Source: CAD feature listing. Evaluate the final solid. Frame: model axes, mm. A direction names the side the tool comes from. Give positions to 0.01 mm unless a question says otherwise; leave off trailing zeros. Order: outer loops, then holes, each group sorted by start corner. A loop starts at its lowest first (then second) coordinate and runs counter-clockwise, first axis right, second up. Notation, with made-up numbers: (36, 33.25) - (57, 33.25) arc R27 ccw to (57, 68.25) - close; hole circle Ø11 at (35.25, -8). An arc over 180 degrees is marked (long way). Answer as CSV lines item,"result".
```python
from build123d import *

# Parameters (mm, degrees)
SKETCH1_R           = 19
SKETCH1_R_2         = 10
BOSS_EXTRUDE1_DEPTH = 20
BOSS_EXTRUDE2_DEPTH = 30
BOSS_EXTRUDE3_DEPTH = 40
SKETCH2_R           = 5
BOSS_EXTRUDE4_DEPTH = 10


with BuildPart() as part:
    # Sketch1 → Boss-Extrude1 (new body)
    with BuildSketch(Plane(origin=(0, 0, 0), x_dir=(0, 0, -1), z_dir=(1, 0, 0))):
        Circle(SKETCH1_R)
        Circle(SKETCH1_R_2, mode=Mode.SUBTRACT)
    extrude(amount=BOSS_EXTRUDE1_DEPTH)

    # Sketch1_3 → Boss-Extrude2 (add)
    with BuildSketch(Plane(origin=(0, 0, 0), x_dir=(0, 0, -1), z_dir=(1, 0, 0))):
        with BuildLine():
            ThreePointArc((-27, 0), (0, -27), (27, 0))
            Line((27, 0), (19, 0))
            ThreePointArc((19, 0), (0, -19), (-19, 0))
            Line((-19, 0), (-27, 0))
        make_face()
    extrude(amount=BOSS_EXTRUDE2_DEPTH)

    # Sketch1_4 → Boss-Extrude3 (add)
    with BuildSketch(Plane(origin=(0, 0, 0), x_dir=(0, 0, -1), z_dir=(1, 0, 0))):
        with BuildLine():
            ThreePointArc((-27, 0), (0, -27), (27, 0))
            Line((27, 0), (36, 0))
            Line((36, 0), (44, -31))
            Line((44, -31), (44, -36))
            Line((44, -36), (38, -36))
            Line((38, -36), (38, -96))
            Line((38, -96), (18, -96))
            Line((18, -96), (18, -76))
            Line((18, -76), (-18, -76))
            Line((-18, -76), (-18, -96))
            Line((-18, -96), (-38, -96))
            Line((-38, -96), (-38, -36))
            Line((-38, -36), (-44, -36))
            Line((-44, -36), (-44, -31))
            Line((-44, -31), (-36, 0))
            Line((-36, 0), (-27, 0))
        make_face()
    extrude(amount=BOSS_EXTRUDE3_DEPTH)

    # Sketch2 → Boss-Extrude4 (add)
    # profile 1 of 2: a face of its own
    with BuildSketch(Plane.XZ.offset(36)):
        with BuildLine():
            Line((10, -63), (10, -42))
            Line((10, -42), (30, -42))
            Line((30, -42), (30, -63))
            ThreePointArc((30, -63), (20, -73), (10, -63))
        make_face()
        with Locations(Location((20, -63, 0), (0, 0, 270))):
            Circle(SKETCH2_R, mode=Mode.SUBTRACT)
    # profile 2 of 2: a face of its own
    with BuildSketch(Plane.XZ.offset(36)):
        with BuildLine():
            Line((30, 42), (30, 63))
            ThreePointArc((30, 63), (20, 73), (10, 63))
            Line((10, 63), (10, 42))
            Line((10, 42), (30, 42))
        make_face()
        with Locations(Location((20, 63, 0), (0, 0, 90))):
            Circle(SKETCH2_R, mode=Mode.SUBTRACT)
    extrude(amount=-BOSS_EXTRUDE4_DEPTH)


solid = part.part
```
(1) Access query for faces 1 (the flat face through (20, 0, 28)), 2 (the flat face through (20, -8, -8)), 3 (the flat face through (20, -76, 0)), 4 (the flat face through (5, -33, -44)), 5 (the flat face through (20, -66, 38)). Directions: +Z, -Z, +X, -X, +Y, -Y. A direction counts if a zero-diameter tool reaches every point of the face in a straight line with its end or side. Return the directions, or none.
Completed:
face 1,"+Z, +X, -X, +Y"
face 2,"+X, +Y"
face 3,"+X, -X, -Y"
face 4,"-Z, -X, +Y, -Y"
face 5,"+Z, +X, -X, -Y"
(2) Cut plane A-A (z = 0). Return loops of the section in (x, y), then the cut area to 3 significant figures.
Completed:
outline,"(0, -76) - (40, -76) - (40, -27) - (30, -27) - (30, -19) - (20, -19) - (20, -10) - (0, -10) - close; (0, 10) - (20, 10) - (20, 19) - (0, 19) - close"
area,"2,560 mm²"
(3) Contact query for flat-ended pins moving along their axis: pin 1 (10 mm diameter, centred on y = -9.5, z = 18.5, fed in from +X); pin 2 (2 mm diameter, centred on x = 10, z = 58, fed in from +Y); pin 3 (18.5 mm diameter, centred on x = 13, z = 26, fed in from +Y). Output: stop coordinate, or through.
Completed:
pin 1,"x = 30"
pin 2,"y = -26"
pin 3,"y = 8.97"
(4) Ray query, line 1 (X direction, y = -31.75, z = 63); line 2 (Y direction, x = 19, z = 0); line 3 (Z direction, x = 34, y = -86). Return the intervals inside material, ascending. Write a range as from..to.
Completed:
line 1,"10..15, 25..30"
line 2,"-76..-10, 10..19"
line 3,"-38..-18, 18..38"
(5) Mould query, pull axis Z, two halves, no side actions, for faces 6 (the cylindrical face through (20, -31, -73)), 7 (the flat face through (20, 0, -27)), 8 (the cylindrical face through (15.12, -31.07, -61.92)). Classes: released by +Z, released by -Z, zero draft, split by the parting line, or undercut.
Completed:
face 6,"released by -Z"
face 7,"zero draft"
face 8,"undercut"
(6) Cut plane C-C (x = 8). Return loops of the section in (y, z).
Completed:
outline,"(-96, -38) - (-36, -38) - (-36, -44) - (-31, -44) - (0, -36) - (0, -19) arc R19 ccw to (0, 19) - (0, 36) - (-31, 44) - (-36, 44) - (-36, 38) - (-96, 38) - (-96, 18) - (-76, 18) - (-76, -18) - (-96, -18) - close; hole circle Ø20 at (0, 0)"
(7) Cut plane B-B (y = -87.5). Return loops of the section in (x, z).
Completed:
outline,"(0, -38) - (40, -38) - (40, -18) - (0, -18) - close; (0, 18) - (40, 18) - (40, 38) - (0, 38) - close"
(8) Cut plane D-D (x = 33.5). Return loops of the section in (y, z).
Completed:
outline,"(-96, -38) - (-36, -38) - (-36, -44) - (-31, -44) - (0, -36) - (0, -27) arc R27 cw to (0, 27) - (0, 36) - (-31, 44) - (-36, 44) - (-36, 38) - (-96, 38) - (-96, 18) - (-76, 18) - (-76, -18) - (-96, -18) - close"
